The model under review builds one solid part; all positions refer to its coordinate system, in mm. A direction names the side the tool comes from. Give positions to 0.01 mm unless a question says otherwise; leave off trailing zeros. Order: outer loops, then holes, each group sorted by start corner. A loop starts at its lowest first (then second) coordinate and runs counter-clockwise, first axis right, second up. Notation, with made-up numbers: (18.5, 5) -> (47.5, 5) arc R20 ccw to (47.5, 35) -> close; hole circle Ø10 at (51, -15.75). An arc over 180 degrees is marked (long way). Use one line per item in the form item = value.
```python
from build123d import *

# Parameters (mm, degrees)
F1_DEPTH = 69.85
F2_SIZE2 = 50.8
F2_SIZE  = 50.8
F4_DEPTH = 19.05


with BuildPart() as f1:
    # F0 (on Right) → F1 (new body, symmetric)
    with BuildSketch(Plane.YZ):
        Polygon((0, 0), (-762, 0), (-762, -139.7), (-139.7, -139.7), (-139.7, -762), (0, -762), align=None)
    extrude(amount=F1_DEPTH, both=True)

    # F2
    f2_edges = [f1.edges().sort_by_distance(p)[0] for p in [
        (0, -762, -139.7),
        (69.85, -69.85, -762),
        (0, -139.7, -762),
        (-69.85, -69.85, -762),
        (0, 0, -762),
        (-69.85, -762, -69.85),
        (0, -762, 0),
        (69.85, -762, -69.85),
    ]]
    chamfer(f2_edges, length=F2_SIZE, length2=F2_SIZE2)

    # F3 (on Right) → F4 (join, symmetric)
    with BuildSketch(Plane.YZ):
        Polygon((-483.876414, -139.7), (-609.6, -139.7), (-139.7, -609.6), (-139.7, -483.876414), align=None)
    extrude(amount=F4_DEPTH, both=True)


solid = f1.part
```
1. Tool access review of faces 4 (the face through (0.267, -309.379, -314.197)), 5 (the face through (1, -120.3, -730.6)), 6 (the face through (-19.05, -341, -339)): name each direction out of +Z, -Z, +X, -X, +Y, -Y from which nothing blocks a thin tool from reaching the whole face with its end or side.
Values:
face_4 = +X, -X
face_5 = -Z, +X, -X, -Y
face_6 = -Z, -X, -Y
2. For L1, parallel to Y at x = 49, z = -642; L2, parallel to Y at x = 11.5, z = -259, list the stretches that pass through material, from the lowest coordinate up.
Values:
L1 = -139.7 to 0
L2 = -490.3 to -364.58, -139.7 to 0
3. For pin 1 Ø4 at (x, z) = (22, -400.5) entering from -Y; pin 2 Ø10 at (x, y) = (27, -345) entering from -Z, all flat-tipped, find the tip position at first contact; note any pin that passes through.
Values:
pin_1 = -139.7
pin_2 = -139.7
4. Add section D-D on y = -222.5. Give the boundary of the cut face in (x, z), then the cut area to 3 significant figures.
Values:
outline = (-69.85, -139.7) -> (69.85, -139.7) -> (69.85, 0) -> (-69.85, 0) -> close; (-19.05, -526.8) -> (19.05, -526.8) -> (19.05, -401.08) -> (-19.05, -401.08) -> close
area = 24,300 mm^2
5. The part is to be moulded in two halves that separate along Y. For faces 1 (the face through (1, -139.7, -421)), 2 (the face through (69.85, -124, -193)), 3 (the face through (-1, -731.3, -20.1)), say which applies: +Y half, -Y half, draft (parallel to the pull), parting line (faces both ways), or undercut.
Values:
face_1 = undercut
face_2 = draft
face_3 = -Y half
6. Add section B-B on z = -392. Give the boundary of the cut face in (x, y).
Values:
outline = (-69.85, -139.7) -> (69.85, -139.7) -> (69.85, 0) -> (-69.85, 0) -> close; (-19.05, -357.3) -> (19.05, -357.3) -> (19.05, -231.58) -> (-19.05, -231.58) -> close
7. Add section C-C on y = -107.5. Give the boundary of the cut face in (x, z), then the cut area to 3 significant figures.
Values:
outline = (-69.85, -711.2) -> (-37.65, -743.4) -> (37.65, -743.4) -> (69.85, -711.2) -> (69.85, 0) -> (-69.85, 0) -> close
area = 103,000 mm^2
8. Add section A-A on x = -32.5. Give the boundary of the cut face in (y, z).
Values:
outline = (-748.55, -102.35) -> (-711.2, -139.7) -> (-139.7, -139.7) -> (-139.7, -711.2) -> (-102.35, -748.55) -> (-37.35, -748.55) -> (0, -711.2) -> (0, 0) -> (-711.2, 0) -> (-748.55, -37.35) -> close
